Solid Edge part; units mm, degrees
sketch "Sketch1" plane through (0, 0, 0) normal (0, -1, 0) x (1, 0, 0)
  circle A0 centre (0, 0) radius 35
extrude "Protrusion1" add sketch "Sketch1" against normal blind 10
sketch "Sketch2" plane through (0, 0, 0) normal (0, -1, 0) x (1, 0, 0)
  circle A0 centre (0, 0) radius 23
extrude "ExtrudedProtrusion_2" add sketch "Sketch2" along normal blind 7
sketch "Sketch3" plane through (0, 0, 13) normal (0, 0, 1) x (1, 0, 0)
  line L0 (0, -7) -> (-36.8229, -7)
  line L1 (-36.8229, -7) -> (-44.194, -13.1851)
  line L2 (-44.194, -13.1851) -> (-44.194, -18.1851)
  line L3 (-44.194, -18.1851) -> (-23, -35.969)
  line L4 (-23, -35.969) -> (0, -35.969)
  line L5 (23, -35.969) -> (0, -35.969)
  line L6 (44.194, -18.1851) -> (23, -35.969)
  line L7 (44.194, -13.1851) -> (44.194, -18.1851)
  line L8 (36.8229, -7) -> (44.194, -13.1851)
  line L9 (0, -7) -> (36.8229, -7)
  dimension "D1" = 44.194
extrude "ExtrudedProtrusion_3" add sketch "Sketch3" against normal blind 4
sketch "Sketch4" plane through (0, -21.4845, 13) normal (0, 0, 1) x (0.766, -0.6428, 0)
  circle A0 centre (-35.2842, -22.0364) radius 1.5
  circle A1 centre (27.8287, 30.9216) radius 1.5
extrude "ExtrudedCutout_1" cut sketch "Sketch4" against normal blind 33.266
fillet "Round_1" radius 2 4 edges at (-44.194, -13.1851, 11) (-44.194, -18.1851, 11) (44.194, -18.1851, 11) (44.194, -13.1851, 11)
mirror "Mirror1" about plane through (0, 0, 0) normal (0, 0, 1) of "ExtrudedProtrusion_3", "ExtrudedCutout_1"
fillet "Round1" radius 2 4 edges at (-44.194, -13.1851, -11) (-44.194, -18.1851, -11) (44.194, -18.1851, -11) (44.194, -13.1851, -11)
sketch "Sketch5" plane through (0, -7, 18) normal (0, -1, 0) x (1, 0, 0)
  line L0 (0, -5) -> (-1, -5)
  line L1 (-1, -5) -> (-1, 1)
  line L2 (-1, 1) -> (0, 1)
  line L3 (1, 1) -> (0, 1)
  line L4 (1, -5) -> (1, 1)
  line L5 (0, -5) -> (1, -5)
extrude "ExtrudedProtrusion_5" add sketch "Sketch5" along normal blind 10
fillet "Round_3" radius 1 5 edges at (-1, -12, 19) (1, -12, 19) (1, -17, 16) (-1, -17, 16) (0, -17, 19)
mirror "Mirror2" about plane through (0, 0, 0) normal (0, 0, 1) of "ExtrudedProtrusion_5"
fillet "Round2" radius 1 5 edges at (-1, -12, -19) (1, -12, -19) (1, -17, -16) (-1, -17, -16) (0, -17, -19)
sketch "Sketch6" plane through (0, 10, 0) normal (0, 1, 0) x (0, 0, 1)
  circle A0 centre (0, 0) radius 15
extrude "ExtrudedCutout_3" cut sketch "Sketch6" against normal blind 10
Can you work these out from the model? Positions are in its coordinate system, mm. A direction names the side the tool comes from. Give positions to 0.01 mm unless a question says otherwise; leave off trailing zeros. Order: outer loops, then holes, each group sorted by start corner. A loop starts at its lowest first (then second) coordinate and runs counter-clockwise, first axis right, second up. Notation, with made-up numbers: M 35.25,-15.5 L 75.25,-15.5 A37 ccw 75.25,20.5 Z; hole C -10,24.5 d6. An arc over 180 degrees is marked long. Use one line per item in the form item = value.
Item 1: If I drill on line 1 along Z through (x, y) = (-33.5, -8); line 2 along Y through (x, z) = (-17.5, 18); line 3 along X through (y, z) = (6.5, 12), over which ranges is the centre line in solid material (lowest first)? Write a range as [from, to].
Values follow:
line_1 = [-13, -9], [9, 13]
line_2 = [0, 10]
line_3 = [-32.88, -9], [9, 32.88]
Item 2: Will these pins go through, and if not, where does the flat tip stop? pin 1 Ø8.5 at (x, y) = (-12.5, -25) entering from -Z; pin 2 Ø10 at (x, y) = (5, -19.5) entering from +Z; pin 3 Ø2.5 at (x, y) = (41.19, -15.69) entering from +Z; pin 4 Ø15 at (x, z) = (-3, -0.5) entering from +Y.
Values follow:
pin_1 = -13
pin_2 = 13
pin_3 = through
pin_4 = 0
Item 3: If we section it at B-B, the plane x = 25: Write out the boundary of the cut face in (y, z), and give its area (3 significant figures).
Values follow:
outline = M -34.29,-13 L -7,-13 L -7,-9 L -34.29,-9 Z; M -34.29,9 L -7,9 L -7,13 L -34.29,13 Z; M 0,-24.49 L 10,-24.49 L 10,24.49 L 0,24.49 Z
area = 708 mm^2
Item 4: If we section it at A-A, the plane z = 0: Write out the boundary of the cut face in (x, y).
Values follow:
outline = M -35,0 L -23,0 L -23,-7 L 23,-7 L 23,0 L 35,0 L 35,10 L 15,10 L 15,0 L -15,0 L -15,10 L -35,10 Z
Item 5: For faces 5 (the flat face through (1, -11, 15)), 6 (the flat face through (-28, -7, -11)), 7 (the flat face through (0, -7, 0)), 8 (the flat face through (28, -7, -11)), 9 (the flat face through (-1, -21, 13)), which set-ups out of +Z, -Z, +X, -X, +Y, -Y let a thin tool reach every point of the face, with its end or its side?
Values follow:
face_5 = +Z, +X, -Y
face_6 = -Z, -X
face_7 = +X, -X, -Y
face_8 = -Z, +X
face_9 = +Z, -Y
Item 6: Thinking about a two-plate mould opening in Y: for faces 1 (the flat face through (0.3, -7, 19.2)), 2 (the cylindrical face through (42.625, -16.136, -11.028)), 3 (the flat face through (1, -21, -13)), 4 (the flat face through (-28, -7, 11)), which applies, pulls with the +Y half, pulls with the -Y half, needs draft (parallel to the pull), parting line crosses it, or undercut?
Values follow:
face_1 = pulls with the -Y half
face_2 = undercut
face_3 = needs draft
face_4 = undercut
Item 7: If we section it at C-C, the plane y = -28: Write out the boundary of the cut face in (x, z).
Values follow:
outline = M -32.5,-13 L 32.5,-13 L 32.5,-9 L -32.5,-9 Z; M -32.5,9 L 32.5,9 L 32.5,13 L -32.5,13 Z
